Verification items for this drawing (mm, ordinates from the low corner). A direction names the side the tool comes from. Coordinates: 2 decimals unless noted, no trailing zeros. Order: outer loops, then holes, each group sorted by start corner. A loop starts at its lowest first (then second) coordinate and runs counter-clockwise, first axis right, second up. Notation, with made-up numbers: (79, 72) -> (134, 72) arc R25 cw to (134, 109) -> close; hole circle Ø7 at (48, -39). An arc over 180 degrees is marked (long way). Write item = value, one per line. Start each with the question number.
1. Cross-section at D-D on y = 13.5. Record the cut outline in (x, z).
2. Cross-section at B-B on x = 27.5. Record the cut outline in (y, z).
3. Go/stop test with a flat-tipped pin: P1, Ø12, axis at x = 41.5, y = 17.5, coming from the -Z side. Record where the tip stops, or that it passes through.
4. Cross-section at A-A on y = 30. Record the cut outline in (x, z).
5. Thickness scan on line 1 along X through (y, z) = (47, 21.5); line 2 along Z through (x, y) = (37, 76); line 3 along Y through (x, z) = (31.5, 34). Record the ranges inside material, lowest first. Write a range as from..to.
6. Set-up check for the marked faces 1, 2 and 3: record each of +Z, -Z, +X, -X, +Y, -Y from which the full face is reachable in a straight line by a thin tool's end or side.
7. Cross-section at C-C on x = 39.5. Record the cut outline in (y, z).
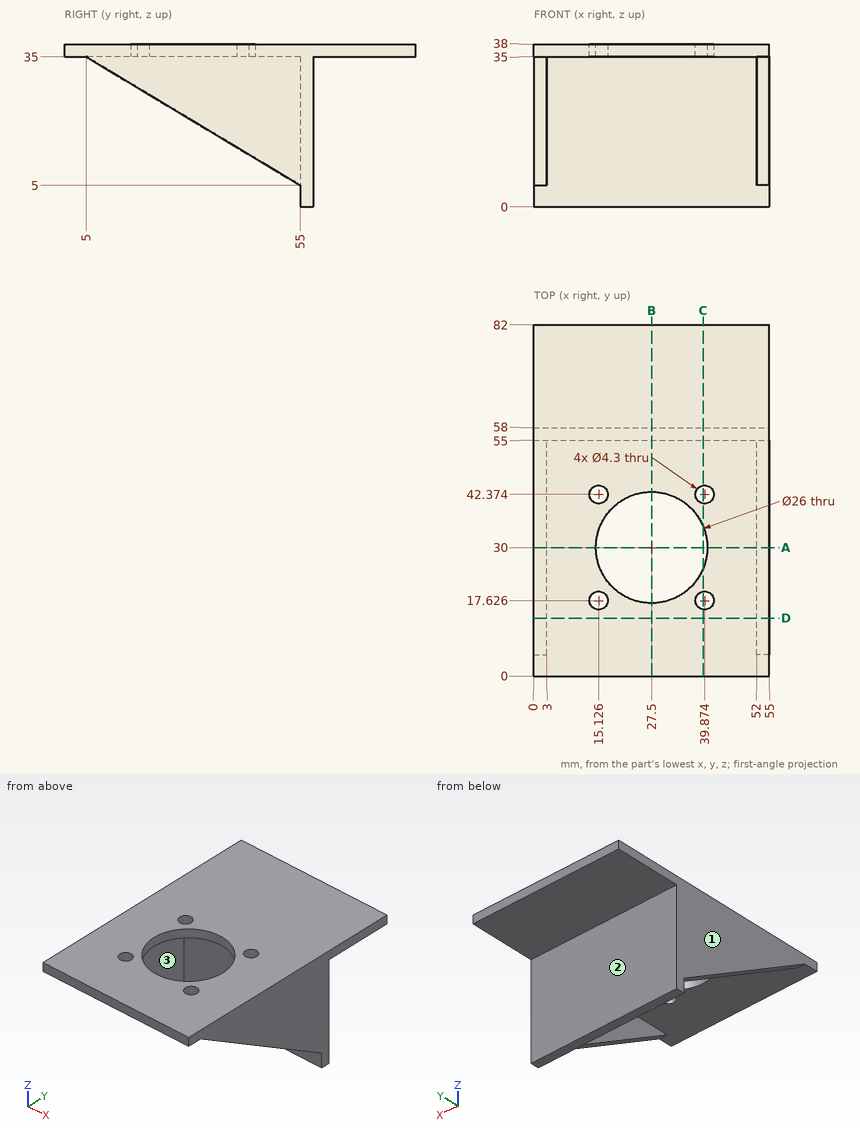
Worked out:
q1.outline = (0, 29.9) -> (3, 29.9) -> (3, 35) -> (52, 35) -> (52, 29.9) -> (55, 29.9) -> (55, 38) -> (0, 38) -> close
q2.outline = (0, 35) -> (17, 35) -> (17, 38) -> (0, 38) -> close; (43, 35) -> (55, 35) -> (55, 0) -> (58, 0) -> (58, 35) -> (82, 35) -> (82, 38) -> (43, 38) -> close
q3.P1 = 35
q4.outline = (0, 20) -> (3, 20) -> (3, 35) -> (14.5, 35) -> (14.5, 38) -> (0, 38) -> close; (40.5, 35) -> (52, 35) -> (52, 20) -> (55, 20) -> (55, 38) -> (40.5, 38) -> close
q5.line_1 = 0..3, 52..55
q5.line_2 = 35..38
q5.line_3 = 55..58
q6.face_1 = +Z, -Z, -X, +Y, -Y
q6.face_2 = -Z, +X, -X, +Y
q6.face_3 = -Z, -Y
q7.outline = (0, 35) -> (15.51, 35) -> (15.51, 38) -> (0, 38) -> close; (19.74, 35) -> (25, 35) -> (25, 38) -> (19.74, 38) -> close; (35, 35) -> (40.26, 35) -> (40.26, 38) -> (35, 38) -> close; (44.49, 35) -> (55, 35) -> (55, 0) -> (58, 0) -> (58, 35) -> (82, 35) -> (82, 38) -> (44.49, 38) -> close
